Autodesk Inventor part; units mm, degrees
ref_plane "YZ Plane" through (0, 0, 0) normal (1, 0, 0) x (0, 1, 0)
ref_plane "XZ Plane" through (0, 0, 0) normal (0, 1, 0) x (-1, 0, 0)
ref_plane "XY Plane" through (0, 0, 0) normal (0, 0, 1) x (1, 0, 0)
sketch "Sketch1" plane through (0, 0, 0) normal (0, 0, 1) x (1, 0, 0)
  line L0 (0, 0) -> (25.4, 0)
  line L1 (25.4, 0) -> (25.4, 50.8)
  line L2 (25.4, 50.8) -> (0, 50.8)
  line L3 (0, 50.8) -> (0, 0)
  line L4 (1.5875, 1.5875) -> (23.8125, 1.5875)
  line L5 (23.8125, 1.5875) -> (23.8125, 49.2125)
  line L6 (23.8125, 49.2125) -> (1.5875, 49.2125)
  line L7 (1.5875, 49.2125) -> (1.5875, 1.5875)
  dimension "d0" = 25.4
  dimension "d1" = 50.8
  dimension "d2" = 1.5875
extrude "Extrusion1" add sketch "Sketch1" along normal blind 685.8
sketch "Sketch2" plane through (0, 50.8, 0) normal (0, 1, 0) x (1, 0, 0)
  line L0 (25.4, 0) -> (0, 0) construction
  line L1 (12.7, 0) -> (12.7, -12.7) construction
  line L2 (12.7, -12.7) -> (12.7, -38.1) construction
  line L3 (0, 0) -> (0, -685.8) construction
  line L4 (0, -342.9) -> (25.4, -342.9) construction
  circle A0 centre (12.7, -38.1) radius 2.5797
  circle A1 centre (12.7, -12.7) radius 2.5797
  line L5 (25.4, -685.8) -> (0, -685.8) construction
  line L6 (12.7, -685.8) -> (12.7, -673.1) construction
  line L7 (12.7, -673.1) -> (12.7, -647.7) construction
  line L8 (0, -685.8) -> (0, 0) construction
  circle A2 centre (12.7, -647.7) radius 2.5797
  circle A3 centre (12.7, -673.1) radius 2.5797
  dimension "d5" = 12.7
  dimension "d6" = 25.4
  dimension "d7" = 5.1594
extrude "Extrusion2" cut sketch "Sketch2" against normal blind 165.1
sketch "Sketch6" plane through (25.4, 0, 0) normal (1, 0, 0) x (0, 0, -1)
  line L0 (0, 50.8) -> (0, 0) construction
  line L1 (0, 25.4) -> (-241.3, 25.4) construction
  line L2 (0, 49.2125) -> (-685.8, 49.2125) construction
  line L3 (-342.9, 49.2125) -> (-342.9, -29.9468) construction
  circle A0 centre (-241.3, 25.4) radius 7.493
  circle A1 centre (-444.5, 25.4) radius 7.493
  dimension "d32" = 241.3
  dimension "d33" = 14.986
extrude "Extrusion9" cut sketch "Sketch6" against normal blind 25.4
sketch "Sketch7" plane through (0, 50.8, 0) normal (0, 1, 0) x (1, 0, 0)
  line L0 (0, 0) -> (0, -83.35) construction
  line L1 (0, 0) -> (0, -685.8) construction
  line L2 (0, -83.35) -> (0, -77) construction
  line L3 (0, -77) -> (4.75, -77) construction
  line L4 (4.75, -77) -> (20.75, -77) construction
  line L5 (20.75, -77) -> (20.75, -63.5) construction
  line L6 (20.75, -63.5) -> (4.75, -63.5) construction
  circle A0 centre (4.75, -77) radius 2.3
  circle A1 centre (4.75, -63.5) radius 2.3
  circle A2 centre (20.75, -63.5) radius 2.3
  circle A3 centre (20.75, -77) radius 2.3
  line L7 (25.4, 0) -> (25.4, -685.8) construction
  line L8 (25.4, -342.9) -> (0, -342.9) construction
  circle A4 centre (4.75, -608.8) radius 2.3
  circle A5 centre (4.75, -622.3) radius 2.3
  circle A6 centre (20.75, -622.3) radius 2.3
  circle A7 centre (20.75, -608.8) radius 2.3
  dimension "d37" = 83.35
  dimension "d38" = 6.35
  dimension "d39" = 4.75
  dimension "d40" = 16
  dimension "d41" = 13.5
  dimension "d42" = 4.6
  dimension "d45" = 4.6
  dimension "d46" = 4.6
  dimension "d47" = 4.6
extrude "Extrusion10" cut sketch "Sketch7" against normal blind 100.0125
properties part number "1x1 27in"
Model file for the job. Use its own axes, mm. A direction names the side the tool comes from. Give positions to 0.01 mm unless a question says otherwise; leave off trailing zeros. Order: outer loops, then holes, each group sorted by start corner. A loop starts at its lowest first (then second) coordinate and runs counter-clockwise, first axis right, second up. Notation, with made-up numbers: (35.25, 9) - (69.25, 9) arc R20 cw to (69.25, 37) - close; hole circle Ø7 at (-10, -13.5). An arc over 180 degrees is marked (long way). One line per item, written item: value.
Item 1: Tool access for faces 4 (the flat face through (13, 50.8, 338)), 5 (the flat face through (13, 1.588, 338)): list every direction of +Z, -Z, +X, -X, +Y, -Y with a clear straight run to the whole face (end or side of a thin tool).
Response values:
face 4: +Z, -Z, +X, -X, +Y
face 5: +Z, -Z
Item 2: Pin check, flat tip, straight feed: pin 1 Ø3.5 at (x, z) = (20.75, 622.3) entering from -Y (3 decimals). Stop position of the tip, or through.
Response values:
pin 1: through
Item 3: Slice it at B-B (z = 444.5). List the corners of the cut face in (x, y), then the cut area to 3 significant figures.
Response values:
outline: (0, 0) - (25.4, 0) - (25.4, 17.91) - (23.81, 17.91) - (23.81, 1.59) - (1.59, 1.59) - (1.59, 17.91) - (0, 17.91) - close; (0, 32.89) - (1.59, 32.89) - (1.59, 49.21) - (23.81, 49.21) - (23.81, 32.89) - (25.4, 32.89) - (25.4, 50.8) - (0, 50.8) - close
area: 184 mm2
Item 4: Slice it at C-C (z = 354). List the corners of the cut face in (x, y).
Response values:
outline: (0, 0) - (25.4, 0) - (25.4, 50.8) - (0, 50.8) - close; hole (1.59, 1.59) - (23.81, 1.59) - (23.81, 49.21) - (1.59, 49.21) - close
Item 5: Two-plate mould, pull along X, no slides. Class faces 1 (the flat face through (23.812, 25, 338)), 2 (the cylindrical face through (24.617, 27.651, 234.153)), 3 (the flat face through (25.4, 25, 338)): released by +X, released by -X, zero draft, split by the parting line, or undercut.
Response values:
face 1: undercut
face 2: zero draft
face 3: released by +X
Item 6: Slice it at A-A (y = 25.4). List the corners of the cut face in (x, z), then the cut area to 3 significant figures.
Response values:
outline: (0, 0) - (1.59, 0) - (1.59, 233.81) - (0, 233.81) - close; (0, 248.79) - (1.59, 248.79) - (1.59, 437.01) - (0, 437.01) - close; (0, 451.99) - (1.59, 451.99) - (1.59, 685.8) - (0, 685.8) - close; (23.81, 0) - (25.4, 0) - (25.4, 233.81) - (23.81, 233.81) - close; (23.81, 248.79) - (25.4, 248.79) - (25.4, 437.01) - (23.81, 437.01) - close; (23.81, 451.99) - (25.4, 451.99) - (25.4, 685.8) - (23.81, 685.8) - close
area: 2,080 mm2
Item 7: Wall check: line 1 (Z direction, x = 12.7, y = 49.95); line 2 (X direction, y = 50, z = 63) (3 decimals); line 3 (X direction, y = 17, z = 159). Give the ranges that are in metal, low to high.
Response values:
line 1: 0 to 10.12, 15.28 to 35.52, 40.68 to 645.12, 650.28 to 670.52, 675.68 to 685.8
line 2: 0 to 2.505, 6.995 to 18.505, 22.995 to 25.4
line 3: 0 to 1.59, 23.81 to 25.4
